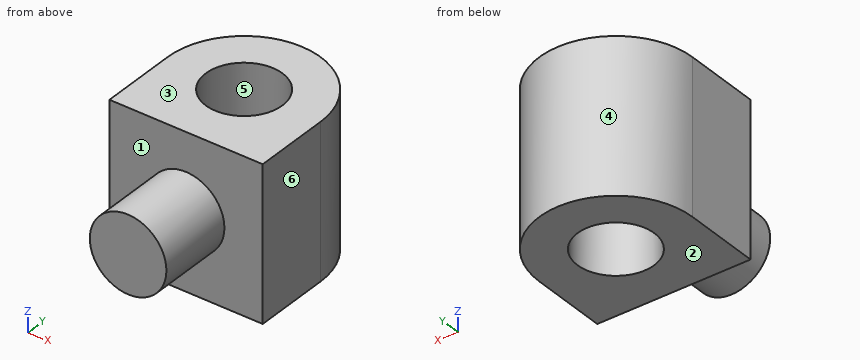
from build123d import *

# Parameters (mm, degrees)
SKETCH1_LINK5_R     = 15
BOSS_EXTRUDE1_DEPTH = 30
SKETCH2_LINK5_R     = 15
BOSS_EXTRUDE2_DEPTH = 30


with BuildPart() as part:
    # sketch1_link5 → Boss-Extrude1 (new body, symmetric)
    with BuildSketch(Plane.XY):
        with BuildLine():
            Line((-30, 0), (-30, -30))
            Line((-30, -30), (30, -30))
            Line((30, -30), (30, 0))
            ThreePointArc((30, 0), (0, 30), (-30, 0))
        make_face()
        Circle(SKETCH1_LINK5_R, mode=Mode.SUBTRACT)
    extrude(amount=BOSS_EXTRUDE1_DEPTH, both=True)

    # sketch2_link5 → Boss-Extrude2 (add)
    with BuildSketch(Plane.XZ.offset(30)):
        Circle(SKETCH2_LINK5_R)
    extrude(amount=BOSS_EXTRUDE2_DEPTH)


solid = part.part
For this review, take the finished solid that the model builds, in its own axes (mm). Face numbers are marked on the shaded views. A direction names the side the tool comes from. Coordinates: 2 decimals unless noted, no trailing zeros. Loops run counter-clockwise (first coordinate to the right, second up) from the corner with the lowest first, then second, coordinate; pieces in that order, holes last. Notation, with made-up numbers: (-35, 3) - (-6, 3) arc R33 cw to (-6, 35) - close; hole circle Ø3 at (7.5, 79). An arc over 180 degrees is marked (long way). Use a Markdown table: item, result. Add a question column.
Item 1: For line 1 (Y direction, x = 0, z = -16.5); line 2 (Y direction, x = 0, z = 12); line 3 (X direction, y = -3.5, z = 17), list the stretches that pass through material, from the lowest coordinate up.
Item 2: We need section B-B (x = 0). Give the boundary of the cut face in (y, z), and give its area (3 significant figures).
Item 3: We need section A-A (z = -12). Give the boundary of the cut face in (x, y), and give its area (3 significant figures).
Item 4: We need section D-D (z = 0). Give the boundary of the cut face in (x, y), and give its area (3 significant figures).
Item 5: Tool access review of the marked faces 1 and 2: name each direction out of +Z, -Z, +X, -X, +Y, -Y from which nothing blocks a thin tool from reaching the whole face with its end or side.
Item 6: Insertion check: pin 1 Ø18 at (x, y) = (0, 0) entering from +Z; pin 2 Ø1 at (y, z) = (-39, -11.5) entering from +X; pin 3 Ø2 at (x, z) = (0.5, -5.5) entering from +Y; pin 4 Ø10 at (y, z) = (-50, -15) entering from -X. Each pin has a flat end and moves straight along its axis. Give the tip position at first contact, or say it passes through.
Item 7: Mouldability with a two-part tool opening along X and no side actions: class the marked faces 3, 4, 5 and 6 as pulls with the +X half, pulls with the -X half, needs draft (parallel to the pull), parting line crosses it, or undercut.
Item 8: We need section C-C (y = 6). Give the boundary of the cut face in (x, z), and give its area (3 significant figures).
Results list:
| question | item | result |
|---|---|---|
| 1 | line 1 | y = -30 to -15, 15 to 30 |
| 1 | line 2 | y = -60 to -15, 15 to 30 |
| 1 | line 3 | x = -30 to -14.59, 14.59 to 30 |
| 2 | outline | (-60, -15) - (-30, -15) - (-30, -30) - (-15, -30) - (-15, 30) - (-30, 30) - (-30, 15) - (-60, 15) - close; (15, -30) - (30, -30) - (30, 30) - (15, 30) - close |
| 2 | area | 2,700 mm^2 |
| 3 | outline | (-30, -30) - (-9, -30) - (-9, -60) - (9, -60) - (9, -30) - (30, -30) - (30, 0) arc R30 ccw to (-30, 0) - close; hole circle Ø30 at (0, 0) |
| 3 | area | 3,050 mm^2 |
| 4 | outline | (-30, -30) - (-15, -30) - (-15, -60) - (15, -60) - (15, -30) - (30, -30) - (30, 0) arc R30 ccw to (-30, 0) - close; hole circle Ø30 at (0, 0) |
| 4 | area | 3,410 mm^2 |
| 5 | face 1 | -Y |
| 5 | face 2 | -Z, +X, -X, +Y, -Y |
| 6 | pin 1 | passes through |
| 6 | pin 2 | stops at x = 10.2 |
| 6 | pin 3 | stops at y = 30 |
| 6 | pin 4 | stops at x = -11.18 |
| 7 | face 3 | needs draft |
| 7 | face 4 | parting line crosses it |
| 7 | face 5 | undercut |
| 7 | face 6 | pulls with the +X half |
| 8 | outline | (-29.39, -30) - (-13.75, -30) - (-13.75, 30) - (-29.39, 30) - close; (13.75, -30) - (29.39, -30) - (29.39, 30) - (13.75, 30) - close |
| 8 | area | 1,880 mm^2 |
